Can you work these out from the model? Positions are in its coordinate system, mm. A direction names the side the tool comes from. Give positions to 0.01 mm unless a question says otherwise; leave off trailing zeros. Order: outer loops, then holes, each group sorted by start corner. A loop starts at its lowest first (then second) coordinate and runs counter-clockwise, first axis right, second up. Notation, with made-up numbers: M 38,0.5 L 73,0.5 A23 ccw 73,23.5 Z; hole C 1,16 d3. An arc over 180 degrees is marked long. Answer as a JSON object with one key per item and string values.
```python
from build123d import *

# Parameters (mm, degrees)
SKETCH1_W           = 100
SKETCH1_H           = 105
BOSS_EXTRUDE1_DEPTH = 2.54
SKETCH2_W           = 100
SKETCH2_H           = 2.54
BOSS_EXTRUDE2_DEPTH = 40
CHAMFER1_SIZE       = 7.62


with BuildPart() as part:
    # Sketch1 → Boss-Extrude1 (new body)
    with BuildSketch(Plane(origin=(0, 0, 0), x_dir=(1, 0, 0), z_dir=(0, 1, 0))):
        Rectangle(SKETCH1_W, SKETCH1_H)
    extrude(amount=BOSS_EXTRUDE1_DEPTH)

    # Sketch2 → Boss-Extrude2 (add)
    with BuildSketch(Plane(origin=(0, 2.54, 0), x_dir=(1, 0, 0), z_dir=(0, 1, 0))):
        with Locations((0, 3.77)):
            Rectangle(SKETCH2_W, SKETCH2_H)
        with Locations((0, -3.77)):
            Rectangle(SKETCH2_W, SKETCH2_H)
    extrude(amount=BOSS_EXTRUDE2_DEPTH)

    # Chamfer1
    chamfer1_edges = [part.edges().sort_by_distance(p)[0] for p in [
        (0, 2.54, -5.04),
        (0, 2.54, 5.04),
    ]]
    chamfer(chamfer1_edges, length=CHAMFER1_SIZE)


solid = part.part
```
1) I want a section at C-C on z = 36. Write out the boundary of the cut face in (x, y), and give its area (3 significant figures).
Results found:
{"outline": "M -50,0 L 50,0 L 50,2.54 L -50,2.54 Z", "area": "254 mm²"}
2) For faces 1 (the face through (50, 12, 4)), 2 (the face through (-1, 26, -5.04)), 3 (the face through (-1, 42.54, 4)), 4 (the face through (-1, 22, 2.5)), 5 (the face through (-1, 2.54, 32)), which set-ups out of +Z, -Z, +X, -X, +Y, -Y let a thin tool reach every point of the face, with its end or its side?
Results found:
{"face 1": "+Z, -Z, +X, +Y, -Y", "face 2": "-Z, +X, -X, +Y", "face 3": "+Z, -Z, +X, -X, +Y", "face 4": "+X, -X, +Y", "face 5": "+Z, +X, -X, +Y"}
3) I want a section at A-A on y = 21.5. Write out the boundary of the cut face in (x, z), and give its area (3 significant figures).
Results found:
{"outline": "M -50,-5.04 L 50,-5.04 L 50,-2.5 L -50,-2.5 Z; M -50,2.5 L 50,2.5 L 50,5.04 L -50,5.04 Z", "area": "508 mm²"}
4) I need wall thicknesses on L1, parallel to Z at x = 21.5, y = 22.5; L2, parallel to Y at x = -36, z = -24; L3, parallel to Z at x = -24.5, y = 10. Which ranges of each line are inside material? Lowest first, please.
Results found:
{"L1": "z = -5.04 to -2.5, 2.5 to 5.04", "L2": "y = 0 to 2.54", "L3": "z = -5.2 to -2.5, 2.5 to 5.2"}
5) I'm going to push flat-ended pins straight in: pin 1 Ø12 at (x, y) = (-14.5, 29.5) entering from -Z; pin 2 Ø5 at (x, y) = (12.5, 15) entering from +Z; pin 3 Ø12 at (x, y) = (15, 13.5) entering from +Z. Where does each tip first touch, or does it pass through?
Results found:
{"pin 1": "stops at z = -5.04", "pin 2": "stops at z = 5.04", "pin 3": "stops at z = 7.7"}
6) Thinking about a two-plate mould opening in Z: for faces 6 (the face through (-1, 26, 5.04)), 7 (the face through (-0.7, 6.4, -8.8)), 8 (the face through (-1, 2.54, -33)), 9 (the face through (-1, 22, -2.5)), which applies, pulls with the +Z half, pulls with the -Z half, needs draft (parallel to the pull), parting line crosses it, or undercut?
Results found:
{"face 6": "pulls with the +Z half", "face 7": "pulls with the -Z half", "face 8": "needs draft", "face 9": "undercut"}
7) I want a section at B-B on x = -39. Write out the boundary of the cut face in (y, z), and give its area (3 significant figures).
Results found:
{"outline": "M 0,-52.5 L 2.54,-52.5 L 2.54,-12.66 L 10.16,-5.04 L 42.54,-5.04 L 42.54,-2.5 L 2.54,-2.5 L 2.54,2.5 L 42.54,2.5 L 42.54,5.04 L 10.16,5.04 L 2.54,12.66 L 2.54,52.5 L 0,52.5 Z", "area": "528 mm²"}
